from build123d import *

# Parameters (mm, degrees)
F1_DEPTH = 2.5
F10_SIZE = 5
F2_W     = 60
F2_H     = 3
F3_DEPTH = 2.5
F4_SIZE  = 10
F5_W     = 1
F5_H     = 2.5
F6_DEPTH = 5
F8_D     = 5


with BuildPart() as f1:
    # F0 (on Front) → F1 (new body)
    with BuildSketch(Plane.XZ):
        Polygon((150, 0), (0, 450), (-150, 0), align=None)
    extrude(amount=F1_DEPTH)

    # F10
    f10_edges = [f1.edges().sort_by_distance(p)[0] for p in [
        (150, -1.25, 0),
        (-150, -1.25, 0),
    ]]
    chamfer(f10_edges, length=F10_SIZE)

    # F2 (on Front) → F3 (join)
    with BuildSketch(Plane.XZ):
        with Locations((-65, -1.5)):
            Rectangle(F2_W, F2_H)
        with Locations((65, -1.5)):
            Rectangle(F2_W, F2_H)
    extrude(amount=F3_DEPTH)

    # F4
    f4_edges = [f1.edges().sort_by_distance(p)[0] for p in [
        (0, -1.25, 450),
    ]]
    chamfer(f4_edges, length=F4_SIZE)

    # F5 (on face) → F6 (cut)
    with BuildSketch(Plane.XY.offset(440.5131670195)):
        with Locations((0, -1.25)):
            Rectangle(F5_W, F5_H)
    extrude(amount=-F6_DEPTH, mode=Mode.SUBTRACT)

    # F8 (through all)
    with Locations(Plane(origin=(0, 0, 0), x_dir=(1, 0, 0), z_dir=(0, 1, 0))):
        with Locations((-131.9634634726, -13), (-105.5707707781, -13), (-79.1780780836, -13), (-52.785385389, -13), (-26.3926926945, -13), (0, -13), (26.3926926945, -13), (52.785385389, -13), (79.1780780836, -13), (105.5707707781, -13), (131.9634634726, -13), (118.7671171253, -52.5890390418), (92.3744244308, -52.5890390418), (-52.785385389, -92.1780780836), (-39.5890390418, -210.9451952089), (39.5890390418, -52.5890390418), (-26.3926926945, -92.1780780836), (-118.7671171253, -52.5890390418), (-13.1963463473, -210.9451952089), (39.5890390418, -131.7671171253), (-65.9817317363, -131.7671171253), (0, -92.1780780836), (13.1963463473, -210.9451952089), (-79.1780780836, -171.3561561671), (-39.5890390418, -131.7671171253), (13.1963463473, -52.5890390418), (-26.3926926945, -250.5342342507), (-39.5890390418, -290.1232732925), (39.5890390418, -210.9451952089), (-52.785385389, -171.3561561671), (-13.1963463473, -131.7671171253), (-105.5707707781, -92.1780780836), (-65.9817317363, -52.5890390418), (0, -250.5342342507), (-92.3744244308, -52.5890390418), (-65.9817317363, -210.9451952089), (-26.3926926945, -171.3561561671), (13.1963463473, -131.7671171253), (26.3926926945, -92.1780780836), (-39.5890390418, -52.5890390418), (-13.1963463473, -290.1232732925), (26.3926926945, -250.5342342507), (0, -171.3561561671), (-92.3744244308, -131.7671171253), (-13.1963463473, -52.5890390418), (13.1963463473, -290.1232732925), (-79.1780780836, -92.1780780836), (26.3926926945, -171.3561561671), (39.5890390418, -290.1232732925), (-52.785385389, -250.5342342507), (65.9817317363, -210.9451952089), (52.785385389, -250.5342342507), (52.785385389, -171.3561561671), (79.1780780836, -171.3561561671), (65.9817317363, -131.7671171253), (52.785385389, -92.1780780836), (79.1780780836, -92.1780780836), (92.3744244308, -131.7671171253), (105.5707707781, -92.1780780836), (65.9817317363, -52.5890390418), (26.3926926945, -329.7123123342), (13.1963463473, -369.301351376), (0, -408.8903904178), (-13.1963463473, -369.301351376), (-26.3926926945, -329.7123123342), (0, -329.7123123342), (26.3926926945, -329.7123123342), (79.1780780836, -171.3561561671), (65.9817317363, -131.7671171253), (52.785385389, -92.1780780836), (79.1780780836, -92.1780780836), (92.3744244308, -131.7671171253), (105.5707707781, -92.1780780836), (92.3744244308, -131.7671171253), (105.5707707781, -92.1780780836)):
            Hole(F8_D / 2)


solid = f1.part
Verification items for the finished model (mm, model axes). Round coordinates to 2 decimals unless told otherwise and drop trailing zeros. Loops run counter-clockwise (first coordinate to the right, second up) from the corner with the lowest first, then second, coordinate; pieces in that order, holes last. Notation, with made-up numbers: (85.25, 33.5) - (135.25, 33.5) arc R17 ccw to (135.25, 44.5) - close; hole circle Ø4 at (10, -33). An arc over 180 degrees is marked (long way). Answer in a Markdown table with one row per item. Add a question column.
Q1. Release check for a two-part mould opening along X. For faces 1 (the face through (76.8, -1.2, 219.6)), 2 (the face through (-74.774, -1.232, 225.679)), 3 (the face through (-2, -2.5, 123)) record: pulls with the +X half, pulls with the -X half, needs draft (parallel to the pull), parting line crosses it, or undercut.
Q2. Material ranges on line 1 (X direction, y = -1.6, z = 369); line 2 (X direction, y = -2, z = 409.5); line 3 (X direction, y = -0.8, z = 340), recorded low to high.
Q3. Section check B-B on z = 67. Enter the section's corners in (x, y), plus the area to 3 significant figures.
Q4. Section check A-A on y = -0.5. State how many separate pieces and enclosed holes the cut face has, plus the area to 3 significant figures.
Q5. Gauge pin test, flat ends, axial feed: pin 1 (8 mm diameter, centred on x = -26.39, z = 250.53, fed in from +Y); pin 2 (1 mm diameter, centred on y = -0.5, z = 373.5, fed in from +X); pin 3 (1.2 mm diameter, centred on x = -2.5, y = -0.5, fed in from -Z). Record the tip position at first contact, or that the pin passes through.
Found:
| question | item | result |
|---|---|---|
| 1 | face 1 | pulls with the +X half |
| 1 | face 2 | pulls with the -X half |
| 1 | face 3 | needs draft |
| 2 | line 1 | x = -27 to -15.68, -10.71 to 10.71, 15.68 to 27 |
| 2 | line 2 | x = -13.5 to -2.42, 2.42 to 13.5 |
| 2 | line 3 | x = -36.67 to 36.67 |
| 3 | outline | (-127.67, -2.5) - (127.67, -2.5) - (127.67, 0) - (-127.67, 0) - close |
| 3 | area | 638 mm² |
| 4 | separate pieces | 1 |
| 4 | enclosed holes | 66 |
| 4 | area | 66,500 mm² |
| 5 | pin 1 | stops at y = 0 |
| 5 | pin 2 | stops at x = 25.67 |
| 5 | pin 3 | stops at z = 0 |
